Build history of the part. All positions in model axes, mm. Give positions to 0.01 mm unless a question says otherwise; leave off trailing zeros. Write each loop counter-clockwise with the first axis right and the second up, starting at its lowest first coordinate (ties: lowest second). Pieces come first, ordered by that corner, then holes.
from build123d import *

# Parameters (mm, degrees)
SKETCH2_W           = 191
SKETCH2_H           = 136
SKETCH2_R           = 1.55
SKETCH2_R_2         = 1.549999948
SKETCH2_R_3         = 1.5
BOSS_EXTRUDE1_DEPTH = 3
SKETCH3_W           = 10
SKETCH3_H           = 3
SKETCH3_W_2         = 21
CUT_EXTRUDE1_DEPTH  = 3
SKETCH4_W           = 3
SKETCH4_H           = 10
SKETCH4_H_2         = 15
CUT_EXTRUDE2_DEPTH  = 3
CUT_EXTRUDE3_REACH  = 5
SKETCH8_R           = 5
CUT_EXTRUDE4_REACH  = 5
SKETCH9_R           = 3


with BuildPart() as part:
    # Sketch2 → Boss-Extrude1 (new body)
    with BuildSketch(Plane.XY):
        with Locations((95.5, 68)):
            Rectangle(SKETCH2_W, SKETCH2_H)
        with Locations((35, 16)):
            Circle(SKETCH2_R, mode=Mode.SUBTRACT)
        with Locations((35, 10)):
            Circle(SKETCH2_R, mode=Mode.SUBTRACT)
        with Locations((24, 46.069195574)):
            Circle(SKETCH2_R, mode=Mode.SUBTRACT)
        with Locations((24, 54.069195574)):
            Circle(SKETCH2_R, mode=Mode.SUBTRACT)
        with Locations((24, 89.930804426)):
            Circle(SKETCH2_R, mode=Mode.SUBTRACT)
        with Locations((35, 120)):
            Circle(SKETCH2_R, mode=Mode.SUBTRACT)
        with Locations((35, 126)):
            Circle(SKETCH2_R, mode=Mode.SUBTRACT)
        with Locations((175.557368355, 35.25)):
            Circle(SKETCH2_R_2, mode=Mode.SUBTRACT)
        with Locations((163, 42.5)):
            Circle(SKETCH2_R_2, mode=Mode.SUBTRACT)
        with Locations((150.442631645, 35.25)):
            Circle(SKETCH2_R_2, mode=Mode.SUBTRACT)
        with Locations((150.442631645, 20.75)):
            Circle(SKETCH2_R_2, mode=Mode.SUBTRACT)
        with Locations((163, 13.5)):
            Circle(SKETCH2_R_2, mode=Mode.SUBTRACT)
        with Locations((175.557368355, 20.75)):
            Circle(SKETCH2_R_2, mode=Mode.SUBTRACT)
        with Locations((18.8, 78.5)):
            Circle(SKETCH2_R_3, mode=Mode.SUBTRACT)
        with Locations((18.8, 26)):
            Circle(SKETCH2_R_3, mode=Mode.SUBTRACT)
        with Locations((119, 73)):
            Circle(SKETCH2_R_3, mode=Mode.SUBTRACT)
        with Locations((119, 25)):
            Circle(SKETCH2_R_3, mode=Mode.SUBTRACT)
    extrude(amount=BOSS_EXTRUDE1_DEPTH)

    # Sketch3 → Cut-Extrude1 (cut)
    with BuildSketch(Plane.XY.offset(3)):
        with Locations((15, 1.5)):
            Rectangle(SKETCH3_W, SKETCH3_H)
        with Locations((35, 1.5)):
            Rectangle(SKETCH3_W, SKETCH3_H)
        with Locations((55, 1.5)):
            Rectangle(SKETCH3_W, SKETCH3_H)
        with Locations((90.5, 1.5)):
            Rectangle(SKETCH3_W_2, SKETCH3_H)
        with Locations((176, 1.5)):
            Rectangle(SKETCH3_W, SKETCH3_H)
        with Locations((156, 1.5)):
            Rectangle(SKETCH3_W, SKETCH3_H)
        with Locations((136, 1.5)):
            Rectangle(SKETCH3_W, SKETCH3_H)
    cut_extrude1 = extrude(amount=-CUT_EXTRUDE1_DEPTH, mode=Mode.SUBTRACT)

    # Mirror1: Cut-Extrude1 across plane
    add(cut_extrude1.mirror(Plane.ZX.offset(68)), mode=Mode.SUBTRACT)

    # Sketch4 → Cut-Extrude2 (cut)
    with BuildSketch(Plane.XY.offset(3)):
        with Locations((1.5, 121)):
            Rectangle(SKETCH4_W, SKETCH4_H)
        with Locations((1.5, 101)):
            Rectangle(SKETCH4_W, SKETCH4_H)
        with Locations((1.5, 81)):
            Rectangle(SKETCH4_W, SKETCH4_H)
        with Locations((1.5, 15)):
            Rectangle(SKETCH4_W, SKETCH4_H)
        with Locations((1.5, 35)):
            Rectangle(SKETCH4_W, SKETCH4_H)
        with Locations((1.5, 57.5)):
            Rectangle(SKETCH4_W, SKETCH4_H_2)
    cut_extrude2 = extrude(amount=-CUT_EXTRUDE2_DEPTH, mode=Mode.SUBTRACT)

    # Mirror2: Cut-Extrude2 across plane
    add(cut_extrude2.mirror(Plane(origin=(95.5, 0, 0), x_dir=(0, 0, 1), z_dir=(1, 0, 0))), mode=Mode.SUBTRACT)

    # Sketch8 → Cut-Extrude3 (cut, up to next)
    with BuildSketch(Plane(origin=(0, 0, 0), x_dir=(-1, 0, 0), z_dir=(0, 0, -1)), mode=Mode.PRIVATE) as cut_extrude3_sk1:
        with Locations((-163, 28)):
            Circle(SKETCH8_R)
    cut_extrude3_tool1 = extrude(cut_extrude3_sk1.sketch, amount=-CUT_EXTRUDE3_REACH, mode=Mode.PRIVATE) & part.part
    add(cut_extrude3_tool1.solids().sort_by_distance((163, 28, 0))[0], mode=Mode.SUBTRACT)

    # Sketch9 → Cut-Extrude4 (cut, up to next)
    with BuildSketch(Plane.XY.offset(3), mode=Mode.PRIVATE) as cut_extrude4_sk1:
        with Locations((85, 68)):
            Circle(SKETCH9_R)
    cut_extrude4_tool1 = extrude(cut_extrude4_sk1.sketch, amount=-CUT_EXTRUDE4_REACH, mode=Mode.PRIVATE) & part.part
    add(cut_extrude4_tool1.solids().sort_by_distance((85, 68, 3))[0], mode=Mode.SUBTRACT)


solid = part.part
(1) Saw through at B-B, the plane z = 1.2. Give the number of separate pieces and of enclosed holes in the cut face, plus the area to 3 significant figures.
(2) Probe line 1 (Y direction, x = 24, z = 1.15); line 2 (Y direction, x = 119, z = 1.55); line 3 (X direction, y = 73, z = 1.85). List the from-to ranges inside material, lowest first.
(3) Saw through at A-A, the plane y = 68. List the corners of the cut face in (x, z), plus the area to 3 significant figures.
(4) Mould opens along X. For faces 1 (the face through (94, 69, 3)), 2 (the face through (167, 25, 1)), 3 (the face through (82.6, 66.2, 1.5)) say: +X half, -X half, draft (parallel to the pull), parting line (faces both ways), or undercut.
Computed values:
1. separate pieces: 1
1. enclosed holes: 19
1. area: 24,900 mm2
2. line 1: y = 0 to 44.52, 47.62 to 52.52, 55.62 to 88.38, 91.48 to 136
2. line 2: y = 0 to 23.5, 26.5 to 71.5, 74.5 to 136
2. line 3: x = 0 to 117.5, 120.5 to 191
3. outline: (0, 0) - (82, 0) - (82, 3) - (0, 3) - close; (88, 0) - (191, 0) - (191, 3) - (88, 3) - close
3. area: 555 mm2
4. face 1: draft
4. face 2: undercut
4. face 3: undercut
